Autodesk Inventor part; units mm, degrees
ref_plane "YZ Plane" through (0, 0, 0) normal (1, 0, 0) x (0, 1, 0)
ref_plane "XZ Plane" through (0, 0, 0) normal (0, 1, 0) x (-1, 0, 0)
ref_plane "XY Plane" through (0, 0, 0) normal (0, 0, 1) x (1, 0, 0)
sketch "Sketch1" plane through (0, 0, 0) normal (1, 0, 0) x (0, 1, 0)
  line L0 (-25, -25) -> (25, -25)
  line L1 (25, -25) -> (25, 25)
  line L2 (25, 25) -> (-25, 25)
  line L3 (-25, 25) -> (-25, -25)
  line L4 (-25, -25) -> (25, 25) construction
  line L5 (25, -25) -> (-25, 25) construction
  line L6 (-24, -24) -> (24, -24)
  line L7 (24, -24) -> (24, 24)
  line L8 (24, 24) -> (-24, 24)
  line L9 (-24, 24) -> (-24, -24)
  line L10 (-24, -24) -> (24, 24) construction
  line L11 (24, -24) -> (-24, 24) construction
  point P0 (0, 0)
  dimension "d0" = 50
  dimension "d1" = 50
  dimension "d2" = 48
  dimension "d3" = 48
extrude "Extrusion1" add sketch "Sketch1" along normal blind 2 contours L3 L2 L1 L0 | L9 L8 L7 L6
sketch "Sketch3" plane through (0, 0, 0) normal (-1, 0, 0) x (0, 0, 1)
  line L0 (19.3, -19.3) -> (-19.3, -19.3)
  line L1 (-19.3, -19.3) -> (-19.3, 19.3)
  line L2 (-19.3, 19.3) -> (19.3, 19.3)
  line L3 (19.3, 19.3) -> (19.3, -19.3)
  line L4 (19.3, -19.3) -> (-19.3, 19.3) construction
  line L5 (-19.3, -19.3) -> (19.3, 19.3) construction
  circle A0 centre (-19.3, 19.3) radius 1.5
  circle A1 centre (19.3, 19.3) radius 1.5555
  circle A2 centre (19.3, -19.3) radius 1.5555
  circle A3 centre (-19.3, -19.3) radius 1.5555
  point P0 (0, 0)
  dimension "d6" = 38.6
  dimension "d7" = 38.6
  dimension "d8" = 3
  dimension "d9" = 3.111
  dimension "d10" = 3.111
  dimension "d11" = 3.111
hole "Hole1" at (0, 19.3, -19.3) direction (1, 0, 0) diameter 3 end through all
sketch "Sketch4" plane through (0, 0, 0) normal (-1, 0, 0) x (0, 0, 1)
  line L0 (-19.3, -19.3) -> (19.3, -19.3)
  line L1 (19.3, -19.3) -> (19.3, 19.3)
  line L2 (19.3, 19.3) -> (-19.3, 19.3)
  line L3 (-19.3, 19.3) -> (-19.3, -19.3)
  line L4 (-19.3, -19.3) -> (19.3, 19.3) construction
  line L5 (19.3, -19.3) -> (-19.3, 19.3) construction
  circle A0 centre (19.3, 19.3) radius 1.5
  point P0 (0, 0)
  dimension "d19" = 38.6
  dimension "d20" = 38.6
  dimension "d21" = 3
hole "Hole2" at (0, 19.3, 19.3) direction (1, 0, 0) diameter 3 end through all
sketch "Sketch5" plane through (0, 0, 0) normal (-1, 0, 0) x (0, 0, 1)
  line L0 (19.3, -19.3) -> (-19.3, -19.3)
  line L1 (-19.3, -19.3) -> (-19.3, 19.3)
  line L2 (-19.3, 19.3) -> (19.3, 19.3)
  line L3 (19.3, 19.3) -> (19.3, -19.3)
  line L4 (19.3, -19.3) -> (-19.3, 19.3) construction
  line L5 (-19.3, -19.3) -> (19.3, 19.3) construction
  circle A0 centre (-19.3, -19.3) radius 1.5
  point P0 (0, 0)
  dimension "d29" = 38.6
  dimension "d30" = 38.6
  dimension "d31" = 3
hole "Hole3" at (0, -19.3, -19.3) direction (1, 0, 0) diameter 3 end through all
sketch "Sketch6" plane through (0, 0, 0) normal (-1, 0, 0) x (0, 0, 1)
  line L0 (19.3, -19.3) -> (-19.3, -19.3)
  line L1 (-19.3, -19.3) -> (-19.3, 19.3)
  line L2 (-19.3, 19.3) -> (19.3, 19.3)
  line L3 (19.3, 19.3) -> (19.3, -19.3)
  line L4 (19.3, -19.3) -> (-19.3, 19.3) construction
  line L5 (-19.3, -19.3) -> (19.3, 19.3) construction
  circle A0 centre (19.3, -19.3) radius 1.5
  point P0 (0, 0)
  dimension "d39" = 38.6
  dimension "d40" = 38.6
  dimension "d41" = 3
hole "Hole4" at (0, -19.3, 19.3) direction (1, 0, 0) diameter 3 end through all
sketch "Sketch7" plane through (0, 0, 0) normal (-1, 0, 0) x (0, 0, 1)
  line L0 (23, -23) -> (-23, -23)
  line L1 (-23, -23) -> (-23, 23)
  line L2 (-23, 23) -> (23, 23)
  line L3 (23, 23) -> (23, -23)
  line L4 (23, -23) -> (-23, 23) construction
  line L5 (-23, -23) -> (23, 23) construction
  line L6 (-25, 25) -> (25, 25)
  line L7 (10, 21) -> (-10, 21)
  line L8 (-10, 21) -> (-10, 25)
  line L9 (-10, 25) -> (10, 25)
  line L10 (10, 25) -> (10, 21)
  line L11 (10, 21) -> (-10, 25) construction
  line L12 (-10, 21) -> (10, 25) construction
  line L13 (21, -10) -> (25, -10)
  line L14 (25, -10) -> (25, 10)
  line L15 (25, 10) -> (21, 10)
  line L16 (21, 10) -> (21, -10)
  line L17 (21, -10) -> (25, 10) construction
  line L18 (25, -10) -> (21, 10) construction
  line L19 (25, -25) -> (-25, -25)
  line L20 (-10, -21) -> (10, -21)
  line L21 (10, -21) -> (10, -25)
  line L22 (10, -25) -> (-10, -25)
  line L23 (-10, -25) -> (-10, -21)
  line L24 (-10, -21) -> (10, -25) construction
  line L25 (10, -21) -> (-10, -25) construction
  line L26 (-25.0252, 10) -> (-20.9748, 10)
  line L27 (-20.9748, 10) -> (-20.9748, -10)
  line L28 (-20.9748, -10) -> (-25.0252, -10)
  line L29 (-25.0252, -10) -> (-25.0252, 10)
  line L30 (-25.0252, 10) -> (-20.9748, -10) construction
  line L31 (-20.9748, 10) -> (-25.0252, -10) construction
  line L32 (25, -25) -> (-25, -25)
  line L33 (-25, -25) -> (-25, 25)
  line L34 (-25, 25) -> (25, 25)
  line L35 (25, 25) -> (25, -25)
  line L36 (25, -25) -> (-25, 25) construction
  line L37 (-25, -25) -> (25, 25) construction
  point P0 (0, 0)
  point P1 (0, 23)
  point P2 (23, 0)
  point P3 (0, -23)
  point P4 (-23, 0)
  point P5 (-10, 23)
  point P6 (10, 23)
  point P7 (23, 10)
  point P8 (23, -10)
  point P9 (10, -23)
  point P10 (-10, -23)
  point P11 (-23, -10)
  point P12 (-23, 10)
  point P13 (10, 25)
  point P14 (-25, 10)
  point P15 (-25, -10)
  point P16 (-10, -25)
  dimension "d49" = 46
  dimension "d50" = 46
  dimension "d51" = 20
  dimension "d52" = 20
  dimension "d53" = 20
  dimension "d54" = 20
extrude "Extrusion3" cut sketch "Sketch7" against normal blind 2 contours L3 L13 L35 L19 L21 L0 | L23 L19 L33 L28 L1 L0 | L3 L2 L10 L6 L35 L15 | L26 L33 L6 L8 L2 L1
sketch "Sketch9" plane through (0, 0, 0) normal (-1, 0, 0) x (0, 0, 1)
  line L0 (10.6, 12.6) -> (-10.6, 12.6)
  line L1 (-12.6, 10.6) -> (-12.6, -10.6)
  line L2 (-10.6, -12.6) -> (10.6, -12.6)
  line L3 (12.6, -10.6) -> (12.6, 10.6)
  line L4 (12.6, 12.6) -> (-12.6, -12.6) construction
  line L5 (-12.6, 12.6) -> (12.6, -12.6) construction
  arc A0 (-12.6, -10.6) -> (-10.6, -12.6) centre (-10.6, -10.6) ccw
  arc A1 (-10.6, 12.6) -> (-12.6, 10.6) centre (-10.6, 10.6) ccw
  arc A2 (12.6, 10.6) -> (10.6, 12.6) centre (10.6, 10.6) ccw
  arc A3 (10.6, -12.6) -> (12.6, -10.6) centre (10.6, -10.6) ccw
  point P0 (0, 0)
  dimension "d62" = 25.2
  dimension "d63" = 25.2
  dimension "d64" = 2
extrude "Extrusion4" cut sketch "Sketch9" against normal blind 2
properties part number "BottomSide"
Geometry check sheet. Reference: the model listing, model coordinates, mm. A direction names the side the tool comes from. Give positions to 0.01 mm unless a question says otherwise; leave off trailing zeros. Order: outer loops, then holes, each group sorted by start corner. A loop starts at its lowest first (then second) coordinate and runs counter-clockwise, first axis right, second up.
1) Cross-section at C-C (x = 0.9). Give the number of separate pieces and of enclosed holes in the cut face, then the cut area to 3 significant figures.
Results are:
separate pieces: 1
enclosed holes: 5
area: 1,620 mm2
2) Tool access check on faces 4 (the flat face through (1, 23, 16)), 5 (the flat face through (1, 24, -10)), 6 (the flat face through (1, -10, 24)), 7 (the flat face through (1, -24, -10)). Record the directions out of +Z, -Z, +X, -X, +Y, -Y that give a thin tool (end or side, any length) a straight path to the whole face; none if there is none.
Results are:
face 4: +Z, +X, -X, +Y
face 5: -Z, +X, -X, +Y
face 6: +Z, +X, -X, -Y
face 7: -Z, +X, -X, -Y
3) Gauge pin test, flat ends, axial feed: pin 1 (2.5 mm diameter, centred on y = -19.3, z = -19.3, fed in from +X); pin 2 (0.6 mm diameter, centred on x = 1, z = -19, fed in from +Y); pin 3 (0.6 mm diameter, centred on x = 1.5, y = 15, fed in from +Z); pin 4 (1 mm diameter, centred on x = 0.5, y = 24, fed in from +Z). Record the tip position at first contact, or that the pin passes through.
Results are:
pin 1: passes through
pin 2: stops at y = 23
pin 3: stops at z = 23
pin 4: stops at z = 10
4) Cross-section at D-D (z = -9). Record the boundary of the cut face in (x, y).
Results are:
outline: (0, -25) - (2, -25) - (2, -12.6) - (0, -12.6) - close; (0, 12.6) - (2, 12.6) - (2, 25) - (0, 25) - close
5) Material ranges on probe 1 along Y at (x, z) = (0.9, -19.3); probe 2 along Y at (x, z) = (1.7, 6), recorded low to high.
Results are:
probe 1: y = -23 to -20.8, -17.8 to 17.8, 20.8 to 23
probe 2: y = -25 to -12.6, 12.6 to 25
6) Cross-section at A-A (y = 19.3). Record the boundary of the cut face in (x, z).
Results are:
outline: (0, -23) - (2, -23) - (2, -20.8) - (0, -20.8) - close; (0, -17.8) - (2, -17.8) - (2, 17.8) - (0, 17.8) - close; (0, 20.8) - (2, 20.8) - (2, 23) - (0, 23) - close
7) Draft check along Y on faces 1 (the cylindrical face through (1.014, -17.836, 18.975)), 2 (the flat face through (1, -23, 17)), 3 (the flat face through (1, 0, 25)). Enter one of: released by +Y, released by -Y, zero draft, split by the parting line, or undercut.
Results are:
face 1: undercut
face 2: released by -Y
face 3: zero draft
